```python
from build123d import *

# Parameters (mm, degrees)
BASE_FLANGE1_DEPTH        = 10
FILLET1_R                 = 3
CORTAR_EXTRUIR1_START     = -1.75
CORTAR_EXTRUIR1_OUTLINE_R = 1.5
CORTAR_EXTRUIR1_DEPTH     = 1.75
CORTAR_EXTRUIR2_REACH     = 20.79
CROQUIS2_R                = 1.5
SCALE1_SCALE              = 0.888888889
CUT_EXTRUDE2_REACH        = 17.649


# Read off the part's stored shape, not the designer's step: Cortar-Extruir1
# Sheet-metal steps are written as plain solids
with BuildPart() as part:
    # Sketch1 → Base-Flange1 (new, symmetric)
    with BuildSketch(Plane(origin=(0, 0, 0), x_dir=(0, 0, -1), z_dir=(1, 0, 0))):
        with BuildLine():
            Line((0, 0), (11.2634, 0))
            ThreePointArc((11.2634, 0), (11.784254855, 0.215745145), (12, 0.7366))
            Line((12, 0.7366), (12, 8))
            Line((12, 8), (13.75, 8))
            Line((13.75, 8), (13.75, 0.7366))
            ThreePointArc((13.75, 0.7366), (13.021691722, -1.021691722), (11.2634, -1.75))
            Line((11.2634, -1.75), (0, -1.75))
            Line((0, -1.75), (0, 0))
        make_face()
    extrude(amount=BASE_FLANGE1_DEPTH, both=True)

    # Fillet1
    fillet1_edges = [part.edges().sort_by_distance(p)[0] for p in [
        (10, -0.875, 0),
        (10, 8, -12.875),
        (-10, -0.875, 0),
        (-10, 8, -12.875),
    ]]
    fillet(fillet1_edges, radius=FILLET1_R)

    # Cortar-Extruir1 outline → Cortar-Extruir1 (cut)
    with BuildSketch(Plane(origin=(0, 0, 0), x_dir=(1, 0, 0), z_dir=(0, 1, 0)).offset(CORTAR_EXTRUIR1_START)):
        with Locations((-6, 3)):
            Circle(CORTAR_EXTRUIR1_OUTLINE_R)
        with Locations((6, 3)):
            Circle(CORTAR_EXTRUIR1_OUTLINE_R)
    extrude(amount=CORTAR_EXTRUIR1_DEPTH, mode=Mode.SUBTRACT)

    # Croquis2 → Cortar-Extruir2 (cut, up to next)
    with BuildSketch(Plane(origin=(0, 0, -13.75), x_dir=(-1, 0, 0), z_dir=(0, 0, -1)), mode=Mode.PRIVATE) as cortar_extruir2_sk1:
        with Locations((0, 4.25)):
            Circle(CROQUIS2_R)
    cortar_extruir2_tool1 = extrude(cortar_extruir2_sk1.sketch, amount=-CORTAR_EXTRUIR2_REACH, mode=Mode.PRIVATE) & part.part
    add(cortar_extruir2_tool1.solids().sort_by_distance((0, 4.25, -13.75))[0], mode=Mode.SUBTRACT)


with BuildPart() as part_1:
    # Scale1: scaled about (0, 0.956325362, -9.128568618)
    add(part.part.scale(SCALE1_SCALE).moved(Location((0, 0.106258374, -1.014285402))))

    # Sketch2 → Cut-Extrude2 (cut, up to next)
    with BuildSketch(Plane.XY.offset(-11.680952069), mode=Mode.PRIVATE) as cut_extrude2_sk1:
        with BuildLine():
            Line((-8.888888889, 4.550702818), (-8.888888889, 0.761013929))
            Line((-8.888888889, 0.761013929), (-8.551720038, 0.761013929))
            ThreePointArc((-8.551720038, 0.761013929), (-5.357621736, 5.42203153), (0, 7.217369485))
            Line((0, 7.217369485), (-6.222222222, 7.217369485))
            ThreePointArc((-6.222222222, 7.217369485), (-8.107840305, 6.436320901), (-8.888888889, 4.550702818))
        make_face()
    cut_extrude2_tool1 = extrude(cut_extrude2_sk1.sketch, amount=-CUT_EXTRUDE2_REACH, mode=Mode.PRIVATE) & part_1.part
    # Sketch2 → Cut-Extrude2 (cut, up to next)
    with BuildSketch(Plane.XY.offset(-11.680952069), mode=Mode.PRIVATE) as cut_extrude2_sk2:
        with BuildLine():
            Line((6.222222222, 7.217369485), (0, 7.217369485))
            ThreePointArc((0, 7.217369485), (5.357621736, 5.42203153), (8.551720038, 0.761013929))
            Line((8.551720038, 0.761013929), (8.888888889, 0.761013929))
            Line((8.888888889, 0.761013929), (8.888888889, 4.550702818))
            ThreePointArc((8.888888889, 4.550702818), (8.107840305, 6.436320901), (6.222222222, 7.217369485))
        make_face()
    cut_extrude2_tool2 = extrude(cut_extrude2_sk2.sketch, amount=-CUT_EXTRUDE2_REACH, mode=Mode.PRIVATE) & part_1.part
    add(cut_extrude2_tool1.solids().sort_by_distance((-6.729341, 5.184457, -11.680952))[0], mode=Mode.SUBTRACT)
    add(cut_extrude2_tool2.solids().sort_by_distance((6.729341, 5.184457, -11.680952))[0], mode=Mode.SUBTRACT)


solid = part_1.part
```
Model file for the job. Use its own axes, mm. A direction names the side the tool comes from. Give positions to 0.01 mm unless a question says otherwise; leave off trailing zeros. Loops run counter-clockwise (first coordinate to the right, second up) from the corner with the lowest first, then second, coordinate; pieces in that order, holes last. Notation, with made-up numbers: (63, 57) - (97, 57) arc R5 ccw to (97, 61) - close; hole circle Ø7 at (6.25, -36). An arc over 180 degrees is marked (long way). One line per item, written item: value. Start each with the question number.
1. Pull direction X, two halves, no side cores. Call faces 1 (the cylindrical face through (6.565, -0.682, -3.17)), 2 (the flat face through (0, 2, -11.681)), 3 (the cylindrical face through (-4.1, -0.68, -3.17)), 4 (the flat face through (8.889, -1, -9)): pulls with the +X half, pulls with the -X half, needs draft (parallel to the pull), parting line crosses it, or undercut.
2. Pin check, flat tips, straight feed: pin 1 (6 mm diameter, centred on x = -1.5, z = -7.5, fed in from +Y); pin 2 (1.5 mm diameter, centred on x = 5.5, y = 3, fed in from +Z); pin 3 (1.5 mm diameter, centred on y = 1.5, z = -9, fed in from -X); pin 4 (1 mm diameter, centred on y = 0.5, z = -3, fed in from +X). Stop position of each tip, or through.
3. Slice it at A-A (y = -0.25). List the corners of the cut face in (x, z).
4. Slice it at C-C (z = -6.25). List the corners of the cut face in (x, y).
5. Slice it at D-D (x = -3.5). List the corners of the cut face in (y, z), plus the area to 3 significant figures.
6. Which spindle directions (+Z, -Z, +X, -X, +Y, -Y) get a long thin tool onto all of the face, cutting with end or side? Do faces 5 (the flat face through (0, 2, -13.237)), 6 (the flat face through (0, 0.106, -6)). Say none if no direction does.
7. Slice it at B-B (x = -7.25). List the corners of the cut face in (y, z).
8. Probe L1, parallel to Y at x = 5.25, z = -8.5; L2, parallel to Z at x = -1, y = 6.5; L3, parallel to Y at x = 0, z = -12.6. List the from-to ranges inside material, lowest first. Write a range as from..to.
Solution:
1. face 1: undercut
1. face 2: needs draft
1. face 3: undercut
1. face 4: pulls with the +X half
2. pin 1: stops at y = 0.11
2. pin 2: stops at z = -11.68
2. pin 3: passes through
2. pin 4: stops at x = 8.86
3. outline: (-8.89, -12.99) - (8.89, -12.99) - (8.89, -3.68) arc R2.67 ccw to (6.22, -1.01) - (-6.22, -1.01) arc R2.67 ccw to (-8.89, -3.68) - close; hole circle Ø2.67 at (-5.33, -3.68); hole circle Ø2.67 at (5.33, -3.68)
4. outline: (-8.89, -1.45) - (8.89, -1.45) - (8.89, 0.11) - (-8.89, 0.11) - close
5. outline: (-1.45, -11.03) arc R2.21 ccw to (0.76, -13.24) - (6.5, -13.24) - (6.5, -11.68) - (0.76, -11.68) arc R0.65 cw to (0.11, -11.03) - (0.11, -1.01) - (-1.45, -1.01) - close
5. area: 28.0 mm^2
6. face 5: -Z, +X, -X, +Y, -Y
6. face 6: +Z, +X, -X, +Y
7. outline: (-1.45, -11.03) arc R2.21 ccw to (0.76, -13.24) - (3.47, -13.24) - (3.47, -11.68) - (0.76, -11.68) arc R0.65 cw to (0.11, -11.03) - (0.11, -1.22) - (-1.45, -1.22) - close
8. L1: y = -1.45..0.11
8. L2: z = -13.24..-11.68
8. L3: y = -0.79..2.55, 5.22..7.22
